Read the model definition and answer for the solid it produces. Units are mm, in the model's axes. Coordinates: 2 decimals unless noted, no trailing zeros. Return JSON: item names as keys, results as strings.
from build123d import *
from OCP.BRepFilletAPI import BRepFilletAPI_MakeChamfer

# Parameters (mm, degrees)
SKETCH2_W                = 4.318
SKETCH2_H                = 2.794
BASE_EXTRUDE_DEPTH       = 7.2898
CHAMFER1_SIZE            = 1.397
CHAMFER1_SIZE2           = 0.246328792
SKETCH3_W                = 2.794
SKETCH3_H                = 1.27
CUT_EXTRUDE1_DEPTH       = 0.508
SKETCH4_W                = 2.794
SKETCH4_H                = 1.27
CUT_EXTRUDE2_DEPTH       = 0.508
SKETCH5_OUTSIDE_W        = 11.073
SKETCH5_OUTSIDE_H        = 8.102
SKETCH5_OUTSIDE_W_2      = 3.302
SKETCH5_OUTSIDE_H_2      = 3.556
CUT_EXTRUDE3_DEPTH       = 0.254
CHAMFER2_SIZE            = 1.397
CHAMFER2_SIZE_2          = 0.246328792
BOSS_EXTRUDE_THIN1_DEPTH = 1.2065
SKETCH7_W                = 1.524
SKETCH7_H                = 0.381
CUT_EXTRUDE4_DEPTH       = 0.508
SKETCH8_W                = 0.762
SKETCH8_H                = 3.825342416
BOSS_EXTRUDE2_DEPTH      = 0.00254


with BuildPart() as part:
    # Sketch2 → Base-Extrude (new body)
    with BuildSketch(Plane(origin=(-0.1524, 0, 0), x_dir=(0, 0, -1), z_dir=(1, 0, 0))):
        with Locations((0, 1.397)):
            Rectangle(SKETCH2_W, SKETCH2_H)
    extrude(amount=BASE_EXTRUDE_DEPTH)

    # Chamfer1: one chamfer whose edges measure the first distance from different faces: ONE call of the kernel's chamfer builder (chamfer() names one face for all edges)
    chamfer1_edges_1 = [part.edges().sort_by_distance(p)[0] for p in [
        (7.1374, 0, 0),
    ]]
    chamfer1_side_1 = [part.faces().sort_by_distance(p)[0] for p in [
        (7.1374, 1.397, 0),
    ]]
    chamfer1_edges_2 = [part.edges().sort_by_distance(p)[0] for p in [
        (-0.1524, 0, 0),
    ]]
    chamfer1_side_2 = [part.faces().sort_by_distance(p)[0] for p in [
        (-0.1524, 1.397, 0),
    ]]
    chamfer1_edges_3 = [part.edges().sort_by_distance(p)[0] for p in [
        (3.4925, 0, -2.159),
    ]]
    chamfer1_side_3 = [part.faces().sort_by_distance(p)[0] for p in [
        (3.4925, 1.397, -2.159),
    ]]
    chamfer1_edges_4 = [part.edges().sort_by_distance(p)[0] for p in [
        (3.4925, 0, 2.159),
    ]]
    chamfer1_side_4 = [part.faces().sort_by_distance(p)[0] for p in [
        (3.4925, 1.397, 2.159),
    ]]
    chamfer1 = BRepFilletAPI_MakeChamfer(part.part.solid().wrapped)
    for e in chamfer1_edges_1:
        chamfer1.Add(CHAMFER1_SIZE, CHAMFER1_SIZE2, e.wrapped, chamfer1_side_1[0].wrapped)  # the first distance lies on this face
    for e in chamfer1_edges_2:
        chamfer1.Add(CHAMFER1_SIZE, CHAMFER1_SIZE2, e.wrapped, chamfer1_side_2[0].wrapped)  # the first distance lies on this face
    for e in chamfer1_edges_3:
        chamfer1.Add(CHAMFER1_SIZE, CHAMFER1_SIZE2, e.wrapped, chamfer1_side_3[0].wrapped)  # the first distance lies on this face
    for e in chamfer1_edges_4:
        chamfer1.Add(CHAMFER1_SIZE, CHAMFER1_SIZE2, e.wrapped, chamfer1_side_4[0].wrapped)  # the first distance lies on this face
    add(Compound.cast(chamfer1.Shape()), mode=Mode.REPLACE)

    # Sketch3 → Cut-Extrude1 (cut)
    with BuildSketch(Plane.ZY.offset(0.1524)):
        with Locations((0, 0.635)):
            Rectangle(SKETCH3_W, SKETCH3_H)
    extrude(amount=-CUT_EXTRUDE1_DEPTH, mode=Mode.SUBTRACT)

    # Sketch4 → Cut-Extrude2 (cut)
    with BuildSketch(Plane(origin=(7.1374, 0, 0), x_dir=(0, 0, -1), z_dir=(1, 0, 0))):
        with Locations((0, 0.635)):
            Rectangle(SKETCH4_W, SKETCH4_H)
    extrude(amount=-CUT_EXTRUDE2_DEPTH, mode=Mode.SUBTRACT)

    # Sketch5 outside → Cut-Extrude3 (cut)
    with BuildSketch(Plane.XZ):
        with Locations((3.4925, 0)):
            Rectangle(SKETCH5_OUTSIDE_W, SKETCH5_OUTSIDE_H)
        with Locations((3.429, 0)):
            Rectangle(SKETCH5_OUTSIDE_W_2, SKETCH5_OUTSIDE_H_2, mode=Mode.SUBTRACT)
    extrude(amount=-CUT_EXTRUDE3_DEPTH, mode=Mode.SUBTRACT)

    # Chamfer2
    chamfer2_edges_1 = [part.edges().sort_by_distance(p)[0] for p in [
        (-0.1524, 2.794, 0),
    ]]
    chamfer2_side_1 = [part.faces().sort_by_distance(p)[0] for p in [
        (-0.1524, 2.789073424, 0),
    ]]
    chamfer2_edges_2 = [part.edges().sort_by_distance(p)[0] for p in [
        (7.1374, 2.794, 0),
    ]]
    chamfer2_side_2 = [part.faces().sort_by_distance(p)[0] for p in [
        (7.132473424, 2.794, 0),
    ]]
    chamfer2_edges_3 = [part.edges().sort_by_distance(p)[0] for p in [
        (3.4925, 2.794, 2.159),
    ]]
    chamfer2_side_3 = [part.faces().sort_by_distance(p)[0] for p in [
        (3.4925, 2.789073424, 2.159),
    ]]
    chamfer2_edges_4 = [part.edges().sort_by_distance(p)[0] for p in [
        (3.4925, 2.794, -2.159),
    ]]
    chamfer2_side_4 = [part.faces().sort_by_distance(p)[0] for p in [
        (3.4925, 2.794, -2.154073424),
    ]]
    chamfer2 = BRepFilletAPI_MakeChamfer(part.part.solid().wrapped)
    for e in chamfer2_edges_1:
        chamfer2.Add(CHAMFER2_SIZE - 0.0001, CHAMFER2_SIZE_2 - 0.0001, e.wrapped, chamfer2_side_1[0].wrapped)
    for e in chamfer2_edges_2:
        chamfer2.Add(CHAMFER2_SIZE_2 - 0.0001, CHAMFER2_SIZE - 0.0001, e.wrapped, chamfer2_side_2[0].wrapped)
    for e in chamfer2_edges_3:
        chamfer2.Add(CHAMFER2_SIZE - 0.0001, CHAMFER2_SIZE_2 - 0.0001, e.wrapped, chamfer2_side_3[0].wrapped)
    for e in chamfer2_edges_4:
        chamfer2.Add(CHAMFER2_SIZE_2 - 0.0001, CHAMFER2_SIZE - 0.0001, e.wrapped, chamfer2_side_4[0].wrapped)
    add(Compound.cast(chamfer2.Shape()), mode=Mode.REPLACE)  # a hair under: the kernel refuses the full size

    # Sketch6 → Boss-Extrude-Thin1 (add, symmetric)
    with BuildSketch(Plane.XY):
        Polygon((0.295515086, 1.267447171), (-0.002552829, 1.267447171), (-0.254, 1.016), (-0.254, 0.254), (0, 0), (1.2954, 0), (1.2954, 0.254), (0.105210245, 0.254), (0, 0.359210245), (0, 0.910789755), (0.102657416, 1.013447171), (0.295515086, 1.013447171), align=None)
    boss_extrude_thin1 = extrude(amount=BOSS_EXTRUDE_THIN1_DEPTH, both=True)

    # Sketch7 → Cut-Extrude4 (cut)
    with BuildSketch(Plane.ZY.offset(0.254)):
        with Locations((0, 1.0795)):
            Rectangle(SKETCH7_W, SKETCH7_H)
    cut_extrude4 = extrude(amount=-CUT_EXTRUDE4_DEPTH, mode=Mode.SUBTRACT)

    # Mirror1: Boss-Extrude-Thin1, Cut-Extrude4 across plane
    add(boss_extrude_thin1.mirror(Plane(origin=(3.4925, 0, 0), x_dir=(0, 0, 1), z_dir=(1, 0, 0))))
    add(cut_extrude4.mirror(Plane(origin=(3.4925, 0, 0), x_dir=(0, 0, 1), z_dir=(1, 0, 0))), mode=Mode.SUBTRACT)

    # Sketch8 → Boss-Extrude2 (add)
    with BuildSketch(Plane(origin=(0, 2.794, 0), x_dir=(-1, 0, 0), z_dir=(0, 1, 0))):
        with Locations((-0.6096, 0)):
            Rectangle(SKETCH8_W, SKETCH8_H)
    extrude(amount=BOSS_EXTRUDE2_DEPTH)


solid = part.part
1. Flat-ended cylindrical pins translate along their axes: pin 1 Ø1 at (y, z) = (2.5, 1.5) entering from +X; pin 2 Ø0.6 at (x, y) = (6, 0.5) entering from -Z. Find the tip coordinate at first contact, or state that the pin passes through.
Taken from the geometry:
{"pin 1": "stops at x = 7.03", "pin 2": "stops at z = -2.05"}
2. Consider L1, parallel to X at y = 0.2, z = 0.5 (3 decimals); L2, parallel to Y at x = 6, z = -1.75; L3, parallel to Y at x = 2.25, z = 0.35. Determine where each line is inside the solid, lowest interval first.
Taken from the geometry:
{"L1": "x = -0.2 to 1.295, 1.778 to 5.08, 5.69 to 7.185", "L2": "y = 0.25 to 2.79", "L3": "y = 0 to 2.79"}
3. For a pull along Y with two mould halves and no side action, classify faces 1 (the face through (0.356, 0.8, 0)), 2 (the face through (4, 2.794, 0)), 3 (the face through (6.629, 0.8, 0)), 4 (the face through (6, 0, 0)) as +Y half, -Y half, draft (parallel to the pull), parting line (faces both ways), or undercut.
Taken from the geometry:
{"face 1": "undercut", "face 2": "+Y half", "face 3": "undercut", "face 4": "-Y half"}
4. The part is cut by section B-B (y = 0.7). Count the separate pieces of the cut face and the enclosed holes in it, then the cut area to 3 significant figures.
Taken from the geometry:
{"separate pieces": "3", "enclosed holes": "0", "area": "27.8 mm2"}
